Design review of the part built by this model. Coordinates are the model's own, in mm. Face numbers are marked on the shaded views. A direction names the side the tool comes from. Coordinates: 2 decimals unless noted, no trailing zeros. Loops run counter-clockwise (first coordinate to the right, second up) from the corner with the lowest first, then second, coordinate; pieces in that order, holes last. Notation, with made-up numbers: (62, -26.75) -> (89, -26.75) arc R31 cw to (89, 2.25) -> close; hole circle Ø7 at (48.25, 52.5). An arc over 180 degrees is marked (long way). Answer as a JSON object with one key per item and string values.
```python
from build123d import *

# Parameters (mm, degrees)
SKETCH1_R           = 1.778
BOSS_EXTRUDE1_DEPTH = 6
CUT_EXTRUDE1_DEPTH  = 3.5
CHAMFER1_SIZE       = 2.54
CHAMFER1_SIZE2      = 5.08


with BuildPart() as part:
    # Sketch1 → Boss-Extrude1 (new body)
    with BuildSketch(Plane(origin=(0, 0, 0), x_dir=(1, 0, 0), z_dir=(0, 1, 0))):
        with BuildLine():
            Line((14.722227154, 13.97), (29.21, 13.97))
            ThreePointArc((29.21, 13.97), (33.700128061, 12.110128061), (35.56, 7.62))
            Line((35.56, 7.62), (35.56, -7.62))
            ThreePointArc((35.56, -7.62), (33.700128061, -12.110128061), (29.21, -13.97))
            Line((29.21, -13.97), (19.176579466, -13.97))
            ThreePointArc((19.176579466, -13.97), (16.831686562, -14.418815604), (14.818265951, -15.701818182))
            ThreePointArc((14.818265951, -15.701818182), (0, -21.59), (-14.818265951, -15.701818182))
            ThreePointArc((-14.818265951, -15.701818182), (-16.831686562, -14.418815604), (-19.176579466, -13.97))
            Line((-19.176579466, -13.97), (-29.21, -13.97))
            ThreePointArc((-29.21, -13.97), (-33.700128061, -12.110128061), (-35.56, -7.62))
            Line((-35.56, -7.62), (-35.56, 7.62))
            ThreePointArc((-35.56, 7.62), (-33.700128061, 12.110128061), (-29.21, 13.97))
            Line((-29.21, 13.97), (-14.722227154, 13.97))
            ThreePointArc((-14.722227154, 13.97), (-13.078726217, 13.753628997), (-11.547227154, 13.119261314))
            Line((-11.547227154, 13.119261314), (-8.995011096, 11.645738686))
            ThreePointArc((-8.995011096, 11.645738686), (-7.463512032, 11.011371003), (-5.820011096, 10.795))
            Line((-5.820011096, 10.795), (5.820011096, 10.795))
            ThreePointArc((5.820011096, 10.795), (7.463512032, 11.011371003), (8.995011096, 11.645738686))
            Line((8.995011096, 11.645738686), (11.547227154, 13.119261314))
            ThreePointArc((11.547227154, 13.119261314), (13.078726217, 13.753628997), (14.722227154, 13.97))
        make_face()
        Circle(SKETCH1_R, mode=Mode.SUBTRACT)
        with BuildLine():
            Line((-23.495, -2.667), (-29.21, -2.667))
            ThreePointArc((-29.21, -2.667), (-31.877, 0), (-29.21, 2.667))
            Line((-29.21, 2.667), (-23.495, 2.667))
            ThreePointArc((-23.495, 2.667), (-20.828, 0), (-23.495, -2.667))
        make_face(mode=Mode.SUBTRACT)
        with BuildLine():
            Line((23.495, 2.667), (29.21, 2.667))
            ThreePointArc((29.21, 2.667), (31.877, 0), (29.21, -2.667))
            Line((29.21, -2.667), (23.495, -2.667))
            ThreePointArc((23.495, -2.667), (20.828, 0), (23.495, 2.667))
        make_face(mode=Mode.SUBTRACT)
        with BuildLine():
            Line((-15.164419162, 6.734455543), (-12.964714637, 5.464455543))
            ThreePointArc((-12.964714637, 5.464455543), (-10.57417018, 6.105), (-11.214714637, 8.495544457))
            Line((-11.214714637, 8.495544457), (-13.414419162, 9.765544457))
            ThreePointArc((-13.414419162, 9.765544457), (-15.804963619, 9.125), (-15.164419162, 6.734455543))
        make_face(mode=Mode.SUBTRACT)
        with BuildLine():
            Line((13.414419162, 9.765544457), (11.214714637, 8.495544457))
            ThreePointArc((11.214714637, 8.495544457), (10.57417018, 6.105), (12.964714637, 5.464455543))
            Line((12.964714637, 5.464455543), (15.164419162, 6.734455543))
            ThreePointArc((15.164419162, 6.734455543), (15.804963619, 9.125), (13.414419162, 9.765544457))
        make_face(mode=Mode.SUBTRACT)
        with BuildLine():
            Line((1.75, -16.5), (1.75, -13.96))
            ThreePointArc((1.75, -13.96), (0, -12.21), (-1.75, -13.96))
            Line((-1.75, -13.96), (-1.75, -16.5))
            ThreePointArc((-1.75, -16.5), (0, -18.25), (1.75, -16.5))
        make_face(mode=Mode.SUBTRACT)
    extrude(amount=BOSS_EXTRUDE1_DEPTH)

    # Sketch5 → Cut-Extrude1 (cut)
    with BuildSketch(Plane(origin=(0, 6, 0), x_dir=(1, 0, 0), z_dir=(0, 1, 0))):
        with BuildLine():
            Line((-3.96875, -13.96), (-3.96875, -16.5))
            ThreePointArc((-3.96875, -16.5), (0, -20.46875), (3.96875, -16.5))
            Line((3.96875, -16.5), (3.96875, -13.96))
            ThreePointArc((3.96875, -13.96), (0, -9.99125), (-3.96875, -13.96))
        make_face()
        with BuildLine():
            Line((12.305044162, 11.687038321), (10.105339637, 10.417038321))
            ThreePointArc((10.105339637, 10.417038321), (8.652676316, 4.995625), (14.074089637, 3.542961679))
            Line((14.074089637, 3.542961679), (16.273794162, 4.812961679))
            ThreePointArc((16.273794162, 4.812961679), (17.726457484, 10.234375), (12.305044162, 11.687038321))
        make_face()
        with BuildLine():
            Line((-12.305044162, 11.687038321), (-10.105339637, 10.417038321))
            ThreePointArc((-10.105339637, 10.417038321), (-8.652676316, 4.995625), (-14.074089637, 3.542961679))
            Line((-14.074089637, 3.542961679), (-16.273794162, 4.812961679))
            ThreePointArc((-16.273794162, 4.812961679), (-17.726457484, 10.234375), (-12.305044162, 11.687038321))
        make_face()
    extrude(amount=-CUT_EXTRUDE1_DEPTH, mode=Mode.SUBTRACT)

    # Chamfer1
    chamfer1_edges = [part.edges().sort_by_distance(p)[0] for p in [
        (-1.778, 6, 0),
    ]]
    chamfer1_side = [part.faces().sort_by_distance(p)[0] for p in [
        (0, 6, 2.195443335),
    ]]
    chamfer(chamfer1_edges, length=CHAMFER1_SIZE, length2=CHAMFER1_SIZE2, reference=chamfer1_side[0])


solid = part.part
```
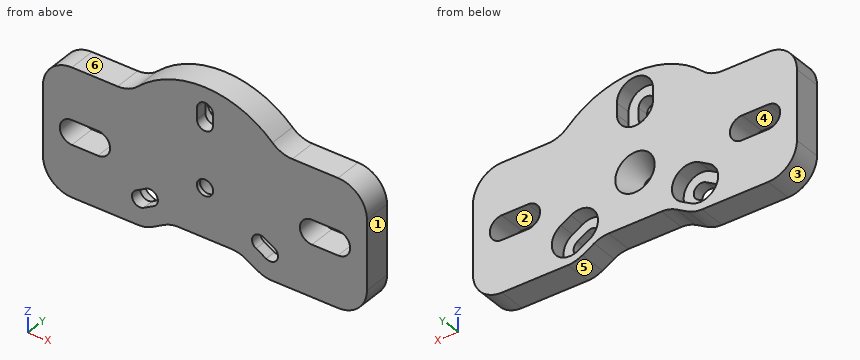
1) Wall thickness on probe 1 along Z at (x, y) = (0, 0.4) (3 decimals); probe 2 along X at (y, z) = (0.4, 0); probe 3 along Z at (x, y) = (-29.5, 0.7): over which ranges is each line inside the solid? List them lowest first.
Completed:
{"probe 1": "-10.795 to -1.778, 1.778 to 12.21, 18.25 to 21.59", "probe 2": "-35.56 to -31.88, -20.83 to -1.78, 1.78 to 20.83, 31.88 to 35.56", "probe 3": "-13.96 to -2.65, 2.65 to 13.96"}
2) Add section B-B, the plane x = 22.5. Give the boundary of the cut face in (y, z).
Completed:
{"outline": "(0, -13.97) -> (6, -13.97) -> (6, -2.47) -> (0, -2.47) -> close; (0, 2.47) -> (6, 2.47) -> (6, 13.97) -> (0, 13.97) -> close"}
3) For the marked faces 4, 5 and 6, list the 3-axis set-ups (+Z, -Z, +X, -X, +Y, -Y) from which the entire face can be reached by the end or side of a thin tool; tool diameter is ignored.
Completed:
{"face 4": "+Y, -Y", "face 5": "-Z, +Y, -Y", "face 6": "+Z, -X, +Y, -Y"}
4) Add section D-D, the plane z = 13. Give the boundary of the cut face in (x, y), and give its area (3 significant figures).
Completed:
{"outline": "(-32.58, 0) -> (-1.46, 0) -> (-1.46, 2.5) -> (-3.85, 2.5) -> (-3.85, 6) -> (-32.58, 6) -> close; (1.46, 0) -> (32.58, 0) -> (32.58, 6) -> (3.85, 6) -> (3.85, 2.5) -> (1.46, 2.5) -> close", "area": "357 mm²"}
5) Add section C-C, the plane x = 0. Give the boundary of the cut face in (y, z) (3 decimals), and give its area (3 significant figures).
Completed:
{"outline": "(0, -10.795) -> (6, -10.795) -> (6, -4.318) -> (0.92, -1.778) -> (0, -1.778) -> close; (0, 1.778) -> (0.92, 1.778) -> (6, 4.318) -> (6, 9.991) -> (2.5, 9.991) -> (2.5, 12.21) -> (0, 12.21) -> close; (0, 18.25) -> (2.5, 18.25) -> (2.5, 20.469) -> (6, 20.469) -> (6, 21.59) -> (0, 21.59) -> close", "area": "108 mm²"}
6) Add section A-A, the plane z = 0. Give the boundary of the cut face in (x, y), and give its area (3 significant figures).
Completed:
{"outline": "(-35.56, 0) -> (-31.88, 0) -> (-31.88, 6) -> (-35.56, 6) -> close; (-20.83, 0) -> (-1.78, 0) -> (-1.78, 0.92) -> (-4.32, 6) -> (-20.83, 6) -> close; (1.78, 0) -> (20.83, 0) -> (20.83, 6) -> (4.32, 6) -> (1.78, 0.92) -> close; (31.88, 0) -> (35.56, 0) -> (35.56, 6) -> (31.88, 6) -> close", "area": "260 mm²"}
7) Clearance check with flat-ended pins moving along their axes: pin 1 Ø3 at (x, y) = (26.5, 2.5) entering from +Z; pin 2 Ø2 at (y, z) = (1.5, 15.5) entering from +X; pin 3 Ø4.5 at (x, z) = (12.5, -7.5) entering from +Y. State where each tip first meets the part, or that it passes through.
Completed:
{"pin 1": "z = 13.97", "pin 2": "x = 16.64", "pin 3": "y = 2.5"}
8) The part is to be moulded in two halves that separate along Z. For the marked faces 1, 2 and 3, say which applies: pulls with the +Z half, pulls with the -Z half, needs draft (parallel to the pull), parting line crosses it, or undercut.
Completed:
{"face 1": "needs draft", "face 2": "undercut", "face 3": "pulls with the -Z half"}
